Autodesk Fusion 360 part; units mm, degrees
sketch "Sketch1" plane through (0, 0, 0) normal (0, 0, 1) x (1, 0, 0)
  line L0 (-3.45, 1.5) -> (-2.25, 1.5)
  line L1 (-2.25, 1.5) -> (-2.25, -1.5)
  line L2 (-2.25, -1.5) -> (-3.45, -1.5)
  line L3 (-3.45, -1.5) -> (-3.45, 1.5)
  line L4 (-5.45, -1.5) -> (-5.45, 1.5) construction
  line L5 (-3.45, 3.5) -> (-2.25, 3.5) construction
  line L6 (-3.45, 3.5) -> (-5.45, 3.5) construction
  line L7 (-5.45, 3.5) -> (-5.45, 1.5) construction
  line L8 (-5.45, 3.5) -> (5.45, 3.5)
  line L9 (5.45, 3.5) -> (5.45, -3.5)
  line L10 (5.45, -3.5) -> (-5.45, -3.5)
  line L11 (-5.45, -3.5) -> (-5.45, 3.5)
  line L12 (0, 1.75) -> (0, 22.5) construction
  line L13 (2.25, 1.5) -> (2.25, -1.5)
  line L14 (2.25, -1.5) -> (3.45, -1.5)
  line L15 (3.45, -1.5) -> (3.45, 1.5)
  line L16 (3.45, 1.5) -> (2.25, 1.5)
  line L17 (1.75, 0) -> (22.5, 0) construction
  dimension "d2" = 1.2
  dimension "d3" = 3
  dimension "d8" = -2
  dimension "d9" = -2
  dimension "d20" = 4.5
  dimension "d21" = 2
  dimension "d22" = 2
  dimension "d23" = 1.5
extrude "Extrude1" add sketch "Sketch1" against normal blind 3.8 draft -0.5 contours L0 L1 L2 L3 | L13 L14 L15 L16 makes body 1 at (-2.2611, 0.4889, -1.2667) makes body 2 at (3.4389, -0.4889, -1.2667)
extrude "Extrude2" add sketch "Sketch1" along normal blind 1 contours L0 L1 L2 L3 | L8 L9 L10 L11 | L13 L14 L15 L16 bodies 1 2
fillet "Fillet1" radius 0.2 4 edges at (-2.2666, 1.4834, -1.9) (-2.2666, -1.4834, -1.9) (-3.4334, 1.4834, -1.9) (-3.4334, -1.4834, -1.9) on bodies 1
fillet "Fillet1" radius 0.25 4 edges at (-2.85, -1.5, 0) (-2.25, 0, 0) (-2.85, 1.5, 0) (-3.45, 0, 0) on bodies 1
fillet "Fillet1" radius 0.2 4 edges at (-2.85, 1.4668, -3.8) (-2.2832, 0, -3.8) (-2.85, -1.4668, -3.8) (-3.4168, 0, -3.8) on bodies 1
fillet "Fillet1" radius 0.2 4 edges at (3.4168, 0, -3.8) (2.2832, 0, -3.8) (2.85, -1.4668, -3.8) (2.85, 1.4668, -3.8) on bodies 1
fillet "Fillet1" radius 0.2 4 edges at (3.4334, -1.4834, -1.9) (2.2666, -1.4834, -1.9) (2.2666, 1.4834, -1.9) (3.4334, 1.4834, -1.9) on bodies 1
fillet "Fillet1" radius 0.25 4 edges at (2.25, 0, 0) (2.85, -1.5, 0) (3.45, 0, 0) (2.85, 1.5, 0) on bodies 1
Input: part model. Units: mm. Frame: model coordinates. Coordinates: 2 decimals unless noted, no trailing zeros. Loops run counter-clockwise (first coordinate to the right, second up) from the corner with the lowest first, then second, coordinate; pieces in that order, holes last. Notation, with made-up numbers: (79.25, -13.75) - (85.25, -13.75) arc R19 cw to (85.25, 23.25) - close; hole circle Ø3 at (75, 26). An arc over 180 degrees is marked (long way). Answer in a Markdown table with one row per item. Add a question column.
Item 1: Mould query, pull axis X, two halves, no side actions, for faces 1 (the flat face through (0, 0, 1)), 2 (the flat face through (-5.45, 0, 0.5)), 3 (the flat face through (0, 0, 0)). Classes: released by +X, released by -X, zero draft, split by the parting line, or undercut.
Item 2: Line query: line 1 along X through (y, z) = (1, -0.3); line 2 along Z through (x, y) = (-4.25, 3); line 3 along Y through (x, z) = (3.25, -0.65). Output: solid intervals per line, ascending. Write a range as [from, to].
Item 3: Section query B-B on x = 1.5. Return the cut outline in (y, z), then the cut area to 3 significant figures.
Item 4: Section query A-A on y = 0. Return the cut outline in (x, z).
Item 5: Section query C-C on y = 2.5. Return the cut outline in (x, z), then the cut area to 3 significant figures.
Recorded:
| question | item | result |
|---|---|---|
| 1 | face 1 | zero draft |
| 1 | face 2 | released by -X |
| 1 | face 3 | undercut |
| 2 | line 1 | [-3.45, -2.25], [2.25, 3.45] |
| 2 | line 2 | [0, 1] |
| 2 | line 3 | [-1.49, 1.49] |
| 3 | outline | (-3.5, 0) - (3.5, 0) - (3.5, 1) - (-3.5, 1) - close |
| 3 | area | 7.00 mm^2 |
| 4 | outline | (-5.45, 0) - (-3.7, 0) arc R0.25 cw to (-3.45, -0.25) - (-3.42, -3.6) arc R0.2 ccw to (-3.22, -3.8) - (-2.48, -3.8) arc R0.2 ccw to (-2.28, -3.6) - (-2.25, -0.25) arc R0.25 cw to (-2, 0) - (2, 0) arc R0.25 cw to (2.25, -0.25) - (2.28, -3.6) arc R0.2 ccw to (2.48, -3.8) - (3.22, -3.8) arc R0.2 ccw to (3.42, -3.6) - (3.45, -0.25) arc R0.25 cw to (3.7, 0) - (5.45, 0) - (5.45, 1) - (-5.45, 1) - close |
| 5 | outline | (-5.45, 0) - (5.45, 0) - (5.45, 1) - (-5.45, 1) - close |
| 5 | area | 10.9 mm^2 |
